```python
from build123d import *

# Parameters (mm, degrees)
F0_R     = 7.85
F1_DEPTH = 25.4
F3_D     = 12.24


# Not quite as in the source:
# - a fillet or chamfer that OpenCascade refuses, or shapes differently, is made with other operations: its cross-section is extruded or revolved along the edge and cut away or added


with BuildPart() as f1:
    # F0 (on Front) → F1 (new body)
    with BuildSketch(Plane.XZ):
        Circle(F0_R)
    extrude(amount=F1_DEPTH)

    # F3 (through all)
    with Locations(Plane(origin=(0, 0, 0), x_dir=(-1, 0, 0), z_dir=(0, 1, 0))):
        with Locations((0, 0)):
            Hole(F3_D / 2)

    # F4: chamfer of 5 on 1 edges, made by hand

    # F4_s1 → F4_t2 (revolve, cut)
    with BuildSketch(Plane.XY):
        Polygon((7.85, -5), (2.85, 0), (7.85, 0), align=None)
    revolve(axis=Axis((0, 0, 0), (0, -1, 0)), mode=Mode.SUBTRACT)

    # F5: chamfer of 5 on 1 edges, made by hand

    # F5_s1 → F5_t2 (revolve, cut)
    with BuildSketch(Plane.XY):
        Polygon((7.85, -20.4), (2.85, -25.4), (7.85, -25.4), align=None)
    revolve(axis=Axis((0, -25.4, 0), (0, -1, 0)), mode=Mode.SUBTRACT)


solid = f1.part
```
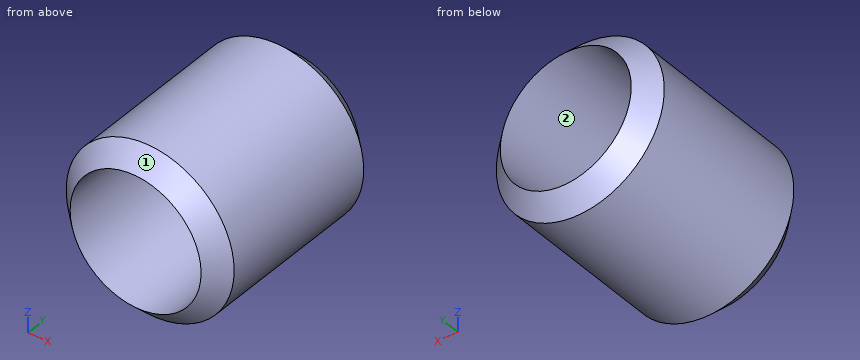
Can you work these out from the model? Positions are in its coordinate system, mm. Face numbers are marked on the shaded views. Round coordinates to 2 decimals unless told otherwise and drop trailing zeros. Order: outer loops, then holes, each group sorted by start corner. A loop starts at its lowest first (then second) coordinate and runs counter-clockwise, first axis right, second up.
(1) If we section it at B-B (x = 0): Please give me the cut outline in (y, z), plus the area to 3 significant figures.
Results are:
outline: (-22.13, -6.12) - (-20.4, -7.85) - (-5, -7.85) - (-3.27, -6.12) - close; (-22.13, 6.12) - (-3.27, 6.12) - (-5, 7.85) - (-20.4, 7.85) - close
area: 59.3 mm2
(2) If we section it at C-C (y = -6.25): Please give me the cut outline in (x, z).
Results are:
outline: circle Ø15.7 at (0, 0); hole circle Ø12.24 at (0, 0)
(3) If we section it at A-A (z = 0): Please give me the cut outline in (x, y).
Results are:
outline: (-7.85, -20.4) - (-6.12, -22.13) - (-6.12, -3.27) - (-7.85, -5) - close; (6.12, -22.13) - (7.85, -20.4) - (7.85, -5) - (6.12, -3.27) - close
(4) I'm going to push flat-ended pins straight in: pin 1 (2 mm diameter, centred on x = 6, y = -8, fed in from -Z); pin 2 (4 mm diameter, centred on y = -14.5, z = 3.5, fed in from +X); pin 3 (6 mm diameter, centred on y = -18, z = -4.5, fed in from -X). Where does each tip first touch, or does it pass through?
Results are:
pin 1: stops at z = -6.05
pin 2: stops at x = 7.71
pin 3: stops at x = -7.71
(5) We'd pull the mould along X, two halves only. Please class the marked faces 1 and 2: +X half, -X half, draft (parallel to the pull), parting line (faces both ways), or undercut.
Results are:
face 1: parting line
face 2: undercut
(6) If I drill on L1, parallel to Z at x = -0.25, y = -14.25; L2, parallel to Z at x = -3, y = -16.25; L3, parallel to X at y = -8.5, z = -4, over which ranges is the centre line in solid material (lowest first)?
Results are:
L1: z = -7.85 to -6.11, 6.11 to 7.85
L2: z = -7.25 to -5.33, 5.33 to 7.25
L3: x = -6.75 to -4.63, 4.63 to 6.75
